For this review, take the finished solid that the model builds, in its own axes (mm). Face numbers are marked on the shaded views. A direction names the side the tool comes from. Give positions to 0.01 mm unless a question says otherwise; leave off trailing zeros. Loops run counter-clockwise (first coordinate to the right, second up) from the corner with the lowest first, then second, coordinate; pieces in that order, holes last.
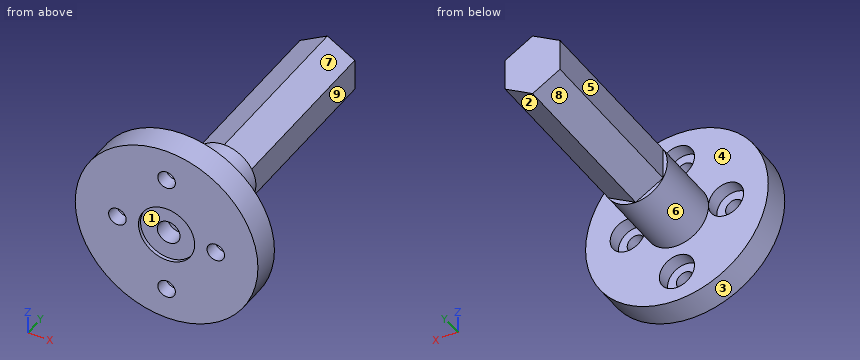
```python
from build123d import *

# Parameters (mm, degrees)
CROQUIS3_R                 = 13
SALIENTE_EXTRUIR1_DEPTH    = 4
CROQUIS4_R                 = 4.5
SALIENTE_EXTRUIR2_DEPTH    = 35
CORTAR_EXTRUIR3_DEPTH      = 44.116122275
CORTAR_EXTRUIR3_DEPTH_BACK = 44.116122275
CROQUIS8_R                 = 1.25
CORTAR_EXTRUIR5_DEPTH      = 40.534794802
CORTAR_EXTRUIR5_DEPTH_BACK = 2
CROQUIS10_R                = 2.5
CROQUIS10_R_2              = 1.25
CROQUIS9_R                 = 1.625
CORTAR_EXTRUIR4_DEPTH      = 3
CROQUIS11_R                = 4
CORTAR_EXTRUIR6_DEPTH      = 0.5
CROQUIS12_OUTSIDE_W        = 38.72
CROQUIS12_OUTSIDE_H        = 38.72
CORTAR_EXTRUIR7_DEPTH      = 25


with BuildPart() as part:
    # Croquis3 → Saliente-Extruir1 (new body)
    with BuildSketch(Plane(origin=(0, 0, 0), x_dir=(1, 0, 0), z_dir=(0, 1, 0))):
        with Locations(Location((0, 0, 0), (0, 0, 270))):
            Circle(CROQUIS3_R)
    extrude(amount=SALIENTE_EXTRUIR1_DEPTH)

    # Croquis4 → Saliente-Extruir2 (add)
    with BuildSketch(Plane(origin=(0, 4, 0), x_dir=(1, 0, 0), z_dir=(0, 1, 0))):
        with Locations(Location((0, 0, 0), (0, 0, 270))):
            Circle(CROQUIS4_R)
    extrude(amount=SALIENTE_EXTRUIR2_DEPTH)

    # Croquis8 → Cortar-Extruir3 (cut, two sides: drawn at the far end of the back side and taken through both)
    with BuildSketch(Plane.XZ.offset(-CORTAR_EXTRUIR3_DEPTH_BACK)):
        with Locations(Location((0, 8.5, 0), (0, 0, 90))):
            Circle(CROQUIS8_R)
        with Locations(Location((0, -8.5, 0), (0, 0, 90))):
            Circle(CROQUIS8_R)
        with Locations(Location((-7, 0, 0), (0, 0, 90))):
            Circle(CROQUIS8_R)
        with Locations(Location((7, 0, 0), (0, 0, 90))):
            Circle(CROQUIS8_R)
    extrude(amount=CORTAR_EXTRUIR3_DEPTH + CORTAR_EXTRUIR3_DEPTH_BACK, mode=Mode.SUBTRACT)

    # Croquis10 → Cortar-Extruir5 (cut, two sides: drawn at the far end of the back side and taken through both)
    # profile 1 of 4: a face of its own
    with BuildSketch(Plane(origin=(0, 4, 0), x_dir=(1, 0, 0), z_dir=(0, 1, 0)).offset(-CORTAR_EXTRUIR5_DEPTH_BACK)):
        with Locations(Location((0, 8.5, 0), (0, 0, 270))):
            Circle(CROQUIS10_R)
    # profile 2 of 4: a face of its own
    with BuildSketch(Plane(origin=(0, 4, 0), x_dir=(1, 0, 0), z_dir=(0, 1, 0)).offset(-CORTAR_EXTRUIR5_DEPTH_BACK)):
        with Locations(Location((0, -8.5, 0), (0, 0, 270))):
            Circle(CROQUIS10_R)
    # profile 3 of 4: a face of its own
    with BuildSketch(Plane(origin=(0, 4, 0), x_dir=(1, 0, 0), z_dir=(0, 1, 0)).offset(-CORTAR_EXTRUIR5_DEPTH_BACK)):
        with Locations(Location((-7, 0, 0), (0, 0, 0.000410889))):
            Circle(CROQUIS10_R)
        with Locations(Location((-7, 0, 0), (0, 0, 270))):
            Circle(CROQUIS10_R_2, mode=Mode.SUBTRACT)
    # profile 4 of 4: a face of its own
    with BuildSketch(Plane(origin=(0, 4, 0), x_dir=(1, 0, 0), z_dir=(0, 1, 0)).offset(-CORTAR_EXTRUIR5_DEPTH_BACK)):
        with Locations(Location((7, 0, 0), (0, 0, 180.000410889))):
            Circle(CROQUIS10_R)
        with Locations(Location((7, 0, 0), (0, 0, 270))):
            Circle(CROQUIS10_R_2, mode=Mode.SUBTRACT)
    extrude(amount=CORTAR_EXTRUIR5_DEPTH + CORTAR_EXTRUIR5_DEPTH_BACK, mode=Mode.SUBTRACT)

    # Croquis9 → Cortar-Extruir4 (cut)
    with BuildSketch(Plane(origin=(0, 0, 0), x_dir=(1, 0, 0), z_dir=(0, 1, 0))):
        with Locations(Location((0, 0, 0), (0, 0, 270))):
            Circle(CROQUIS9_R)
    extrude(amount=CORTAR_EXTRUIR4_DEPTH, mode=Mode.SUBTRACT)

    # Croquis11 → Cortar-Extruir6 (cut)
    with BuildSketch(Plane.XZ):
        with Locations(Location((0, 0, 0), (0, 0, 270))):
            Circle(CROQUIS11_R)
    extrude(amount=-CORTAR_EXTRUIR6_DEPTH, mode=Mode.SUBTRACT)

    # Croquis12 outside → Cortar-Extruir7 (cut)
    with BuildSketch(Plane(origin=(0, 39, 0), x_dir=(1, 0, 0), z_dir=(0, 1, 0))):
        Rectangle(CROQUIS12_OUTSIDE_W, CROQUIS12_OUTSIDE_H)
        Polygon((0, 4.5), (-3.897114317, 2.25), (-3.897114317, -2.25), (0, -4.5), (3.897114317, -2.25), (3.897114317, 2.25), align=None, mode=Mode.SUBTRACT)
    extrude(amount=-CORTAR_EXTRUIR7_DEPTH, mode=Mode.SUBTRACT)


solid = part.part
```
Item 1: Take a section at C-C on x = 7.5. Give the boundary of the cut face in (y, z).
Answer:
outline: (0, -10.62) - (4, -10.62) - (4, -2.45) - (2, -2.45) - (2, -1.15) - (0, -1.15) - close; (0, 1.15) - (2, 1.15) - (2, 2.45) - (4, 2.45) - (4, 10.62) - (0, 10.62) - close
Item 2: Take a section at D-D on y = 23. Give the boundary of the cut face in (x, z).
Answer:
outline: (-3.9, -2.25) - (0, -4.5) - (3.9, -2.25) - (3.9, 2.25) - (0, 4.5) - (-3.9, 2.25) - close
Item 3: For L1, parallel to X at y = 1.1, z = 0 (3 decimals); L2, parallel to X at y = 0.4, z = 0; L3, parallel to X at y = 3.4, z = 0, list the stretches that pass through material, from the lowest coordinate up.
Answer:
L1: x = -13 to -8.25, -5.75 to -1.625, 1.625 to 5.75, 8.25 to 13
L2: x = -13 to -8.25, -5.75 to -4, 4 to 5.75, 8.25 to 13
L3: x = -13 to -9.5, -4.5 to 4.5, 9.5 to 13
Item 4: Clearance check with flat-ended pins moving along their axes: pin 1 Ø1.1 at (x, z) = (-3, 4) entering from +Y; pin 2 Ø12 at (x, y) = (6.5, 19) entering from -Z; pin 3 Ø1.5 at (x, z) = (-1, -8.5) entering from +Y; pin 4 Ø1.5 at (y, z) = (16, -6.5) entering from -X. State where each tip first meets the part, or that it passes through.
Answer:
pin 1: stops at y = 14
pin 2: stops at z = -4.21
pin 3: stops at y = 2
pin 4: passes through
Item 5: Take a section at A-A on z = -9.25. Give the boundary of the cut face in (x, y).
Answer:
outline: (-9.13, 0) - (-1, 0) - (-1, 2) - (-2.38, 2) - (-2.38, 4) - (-9.13, 4) - close; (1, 0) - (9.13, 0) - (9.13, 4) - (2.38, 4) - (2.38, 2) - (1, 2) - close
Item 6: The part is to be moulded in two halves that separate along Z. For the marked faces 1, 2, 3 and 4, say which applies: released by +Z, released by -Z, zero draft, split by the parting line, or undercut.
Answer:
face 1: undercut
face 2: released by -Z
face 3: split by the parting line
face 4: zero draft
Item 7: Tool access review of the marked faces 5, 6, 7, 8 and 9: name each direction out of +Z, -Z, +X, -X, +Y, -Y from which nothing blocks a thin tool from reaching the whole face with its end or side.
Answer:
face 5: +Z, -Z, -X, +Y
face 6: +Y
face 7: +Z, +X, +Y
face 8: -Z, -X, +Y
face 9: +Z, -Z, +X, +Y
Item 8: Take a section at B-B on x = -5. Give the boundary of the cut face in (y, z), and give its area (3 significant figures).
Answer:
outline: (0, -12) - (4, -12) - (4, -1.5) - (2, -1.5) - (2, 1.5) - (4, 1.5) - (4, 12) - (0, 12) - close
area: 90.0 mm2
